Design review of the part built by this model. Coordinates are the model's own, in mm. A direction names the side the tool comes from. Round coordinates to 2 decimals unless told otherwise and drop trailing zeros. Write each loop counter-clockwise with the first axis right and the second up, starting at its lowest first coordinate (ties: lowest second). Pieces come first, ordered by that corner, then holes. Notation, with made-up numbers: M -25,17.25 L -16,17.25 A5 cw -16,23.25 Z; hole C 65,59 d11. An arc over 180 degrees is marked long. One line per question, with ' | ' between items. Start each with the question number.
Item 1: For L1, parallel to Y at x = -69.4, z = 7.75; L2, parallel to X at y = 15, z = 5.5; L3, parallel to Y at x = -69.4, z = 4, list the stretches that pass through material, from the lowest coordinate up.
Item 2: Add section B-B, the plane y = 30.8. State the section outline as (x, z) points, and give its area (3 significant figures).
Item 3: Insertion check: pin 1 Ø11 at (x, y) = (-46, 21) entering from -Z; pin 2 Ø2 at (x, z) = (-47, 9.5) entering from -Y; pin 3 Ø1 at (x, z) = (-60.5, 5.5) entering from -Y. Each pin has a flat end and moves straight along its axis. Give the tip position at first contact, or say it passes through.
Item 4: Machinability: for faces 4 (the face through (-49, 5, 13)), 5 (the face through (-66.231, -31, 7)), 6 (the face through (-38, 14.75, 5)), 7 (the face through (-61, 26.3, 11)), which of the approach directions +Z, -Z, +X, -X, +Y, -Y give a long, thin tool a straight path to every point of the face, cutting with its end or side? Answer none if there is none.
Item 5: Add section A-A, the plane y = -21. State the section outline as (x, z) points, and give its area (3 significant figures).
Item 6: Add section D-D, the plane z = 0.5. State the section outline as (x, y) points, and give its area (3 significant figures).
Item 7: Draft analysis for pull direction X (two halves, no side actions). For faces 1 (the face through (-70, 13.5, 3)), 2 (the face through (-46.05, 13.76, 0.27)), 3 (the face through (-52, 26, 7.5)), state which applies: released by +X, released by -X, zero draft, split by the parting line, or undercut.
Item 8: Add section C-C, the plane x = -47.5. State the section outline as (y, z) points.
```python
from build123d import *

# Parameters (mm, degrees)
SKETCH009_W     = 40
SKETCH009_H     = 69
SKETCH009_R     = 1.75
SKETCH009_W_2   = 31.3
SKETCH009_H_2   = 57.6
PAD004_DEPTH    = 11
SKETCH010_W     = 28
SKETCH010_H     = 23
POCKET005_DEPTH = 8
SKETCH011_W     = 28
SKETCH011_H     = 5
POCKET006_DEPTH = 8
SKETCH012_W     = 25
SKETCH012_H     = 3
POCKET007_DEPTH = 7
SKETCH013_W     = 38
SKETCH013_H     = 5.5
POCKET008_DEPTH = 5
SKETCH014_W     = 31.3
SKETCH014_H     = 2
PAD005_DEPTH    = 11
SKETCH015_W     = 12.5
SKETCH015_H     = 3
POCKET009_DEPTH = 5
SKETCH016_W     = 38
SKETCH016_H     = 5.5
POCKET010_DEPTH = 23.5
PAD006_DEPTH    = 23.5
SKETCH018_W     = 1.2
SKETCH018_H     = 38
PAD007_DEPTH    = 4.3
SKETCH019_W     = 12.15
SKETCH019_H     = 26
PAD008_DEPTH    = 1.2
SKETCH032_W     = 2.35
SKETCH032_H     = 7
POCKET014_DEPTH = 13
SKETCH033_W     = 31.3
SKETCH033_H     = 5
PAD018_DEPTH    = 1.2
SKETCH034_R     = 12
SKETCH034_R_2   = 11
PAD019_DEPTH    = 5.5
PAD020_DEPTH    = 3.5
FILLET_R        = 3
FILLET001_R     = 1


with BuildPart() as part:
    # Sketch009 → Pad004 (new body)
    with BuildSketch(Plane.XY):
        with Locations((-0.1, -1)):
            Rectangle(SKETCH009_W, SKETCH009_H)
        with Locations((-17.5, -32.71)):
            Circle(SKETCH009_R, mode=Mode.SUBTRACT)
        with Locations((17.5, -32.71)):
            Circle(SKETCH009_R, mode=Mode.SUBTRACT)
        with Locations((-17.5, 29.8)):
            Circle(SKETCH009_R, mode=Mode.SUBTRACT)
        with Locations((17.5, 29.8)):
            Circle(SKETCH009_R, mode=Mode.SUBTRACT)
        with Locations((-0.1, -1)):
            Rectangle(SKETCH009_W_2, SKETCH009_H_2, mode=Mode.SUBTRACT)
    extrude(amount=PAD004_DEPTH)

    # Sketch010 (on Face3 of Pad004) → Pocket005 (cut)
    with BuildSketch(Plane.XZ.offset(35.5)):
        with Locations((-0.331047, 5.882488)):
            Rectangle(SKETCH010_W, SKETCH010_H)
    extrude(amount=-POCKET005_DEPTH, mode=Mode.SUBTRACT)

    # Sketch011 (on Face1 of Pocket005) → Pocket006 (cut)
    with BuildSketch(Plane(origin=(0, 33.5, 0), x_dir=(-1, 0, 0), z_dir=(0, 1, 0))):
        with Locations((0, 2.5)):
            Rectangle(SKETCH011_W, SKETCH011_H)
    extrude(amount=-POCKET006_DEPTH, mode=Mode.SUBTRACT)

    # Sketch012 (on Face9 of Pocket006) → Pocket007 (cut)
    with BuildSketch(Plane(origin=(-20.1, 0, 0), x_dir=(0, -1, 0), z_dir=(-1, 0, 0))):
        with Locations((0, 1.5)):
            Rectangle(SKETCH012_W, SKETCH012_H)
    extrude(amount=-POCKET007_DEPTH, mode=Mode.SUBTRACT)

    # Sketch013 (on Face9 of Pocket007) → Pocket008 (cut)
    with BuildSketch(Plane(origin=(-20.1, 0, 0), x_dir=(0, -1, 0), z_dir=(-1, 0, 0))):
        with Locations((-7.5, 8.25)):
            Rectangle(SKETCH013_W, SKETCH013_H)
    extrude(amount=-POCKET008_DEPTH, mode=Mode.SUBTRACT)

    # Sketch014 → Pad005 (join)
    with BuildSketch(Plane.XY):
        with Locations((-0.1, 12.75)):
            Rectangle(SKETCH014_W, SKETCH014_H)
    extrude(amount=PAD005_DEPTH)

    # Sketch015 (on Face9 of Pad005) → Pocket009 (cut)
    with BuildSketch(Plane(origin=(-20.1, 0, 0), x_dir=(0, -1, 0), z_dir=(-1, 0, 0))):
        with Locations((-6.25, 1.5)):
            Rectangle(SKETCH015_W, SKETCH015_H)
    extrude(amount=-POCKET009_DEPTH, mode=Mode.SUBTRACT)

    # Sketch016 (on Face9 of Pocket009) → Pocket010 (cut)
    with BuildSketch(Plane(origin=(-20.1, 0, 0), x_dir=(0, -1, 0), z_dir=(-1, 0, 0))):
        with Locations((-7.5, 8.25)):
            Rectangle(SKETCH016_W, SKETCH016_H)
    extrude(amount=-POCKET010_DEPTH, mode=Mode.SUBTRACT)

    # Sketch017 (on Face9 of Pocket010) → Pad006 (join)
    with BuildSketch(Plane(origin=(-20.1, 0, 0), x_dir=(0, -1, 0), z_dir=(-1, 0, 0))):
        Polygon((11.5, 11), (11.5, 5.5), (-26.5, 5.5), (-26.5, 11), (-25.3, 11), (-25.3, 6.7), (10.3, 6.7), (10.3, 11), align=None)
    extrude(amount=-PAD006_DEPTH)

    # Sketch018 (on Face45 of Pad006) → Pad007 (join)
    with BuildSketch(Plane.XY.offset(6.7)):
        with Locations((2.8, 7.5)):
            Rectangle(SKETCH018_W, SKETCH018_H)
    extrude(amount=PAD007_DEPTH)

    # Sketch019 (on Face36 of Pad007) → Pad008 (join)
    with BuildSketch(Plane(origin=(0, 0, 5.5), x_dir=(1, 0, 0), z_dir=(0, 0, -1))):
        with Locations((9.475, -13.5)):
            Rectangle(SKETCH019_W, SKETCH019_H)
    extrude(amount=-PAD008_DEPTH)

    # Sketch032 (on Face6 of Pad008) → Pocket014 (cut)
    with BuildSketch(Plane(origin=(0, 0, 0), x_dir=(1, 0, 0), z_dir=(0, 0, -1))):
        with Locations((16.725, 26.3)):
            Rectangle(SKETCH032_W, SKETCH032_H)
        with BuildLine():
            ThreePointArc((16.553467, 36.082636), (14.040903, 33.26249), (15.55, 29.8))
            Line((15.55, 29.8), (10.188963, 29.8))
            Line((10.188963, 29.8), (10.188963, 36.082636))
            Line((10.188963, 36.082636), (16.553467, 36.082636))
        make_face()
    extrude(amount=-POCKET014_DEPTH, mode=Mode.SUBTRACT)

    # Sketch033 (on Face43 of Pocket014) → Pad018 (join)
    with BuildSketch(Plane(origin=(0, 0, 5.5), x_dir=(1, 0, 0), z_dir=(0, 0, -1))):
        with Locations((-0.1, -25.3)):
            Rectangle(SKETCH033_W, SKETCH033_H)
    extrude(amount=-PAD018_DEPTH)

    # Sketch034 (on Face41 of Pad018) → Pad019 (join)
    with BuildSketch(Plane(origin=(0, 0, 5.5), x_dir=(1, 0, 0), z_dir=(0, 0, -1))):
        with Locations((-0.15, -12.83)):
            Circle(SKETCH034_R)
        with Locations((-0.15, -12.83)):
            Circle(SKETCH034_R_2, mode=Mode.SUBTRACT)
    extrude(amount=PAD019_DEPTH)

    # Sketch035 (on Face75 of Pad019) → Pad020 (join)
    with BuildSketch(Plane(origin=(0, 0, 0), x_dir=(1, 0, 0), z_dir=(0, 0, -1))):
        with BuildLine():
            ThreePointArc((-6.052, -11.75), (-6.149451, -12.748865), (-6.079047, -13.75))
            Line((-6.079047, -13.75), (5.779047, -13.75))
            ThreePointArc((5.779047, -13.75), (5.849451, -12.748865), (5.752, -11.75))
            Line((-6.052, -11.75), (5.752, -11.75))
        make_face()
    extrude(amount=PAD020_DEPTH)

    # Fillet
    fillet_edges = [part.edges().sort_by_distance(p)[0] for p in [
        (-14.331047, -35.5, 5.5),
    ]]
    fillet(fillet_edges, radius=FILLET_R)

    # Fillet001
    fillet001_edges = [part.edges().sort_by_distance(p)[0] for p in [
        (-14.331047, -29.8, 5.5),
    ]]
    fillet(fillet001_edges, radius=FILLET001_R)


with BuildPart() as part_1:
    # Body001 placement: moved
    add(part.part.moved(Location((-51.9, 1, 2))))


solid = part_1.part
```
Computed values:
1) L1: y = -34.5 to -33.46, -29.96 to 29.05, 32.55 to 34.5 | L2: x = -72 to -67.65, -63.99 to -62.99, -41.11 to -40.11, -36.35 to -32 | L3: y = -34.5 to -33.46, -29.96 to -11.5, 13.5 to 29.05, 32.55 to 34.5
2) outline: M -72,2 L -71.15,2 L -71.15,13 L -72,13 Z; M -67.65,2 L -65.9,2 L -65.9,7 L -37.9,7 L -37.9,2 L -36.15,2 L -36.15,13 L -67.65,13 Z; M -32.65,2 L -32,2 L -32,13 L -32.65,13 Z | area: 223 mm^2
3) pin 1: stops at z = 2 | pin 2: stops at y = 1.5 | pin 3: stops at y = 4.84
4) face 4: +Z, +X, -X, +Y, -Y | face 5: +Z, -Z, -Y | face 6: -Z | face 7: +Z, -X
5) outline: M -72,2 L -67.65,2 L -67.65,13 L -72,13 Z; M -36.35,2 L -32,2 L -32,13 L -36.35,13 Z | area: 95.7 mm^2
6) outline: M -57.98,14.75 A6 ccw -57.95,12.75 L -46.15,12.75 A6 ccw -46.12,14.75 Z | area: 23.9 mm^2
7) face 1: zero draft | face 2: released by +X | face 3: undercut
8) outline: M 1.5,7.5 L 2.73,7.5 L 2.73,2 L 3.82,2 L 3.82,7.5 L 12.75,7.5 L 12.75,-1.5 L 14.75,-1.5 L 14.75,7.5 L 23.84,7.5 L 23.84,2 L 24.93,2 L 24.93,7.5 L 28.8,7.5 L 28.8,7 L 34.5,7 L 34.5,13 L 28.8,13 L 28.8,8.7 L 14.75,8.7 L 14.75,13 L 12.75,13 L 12.75,8.7 L 1.5,8.7 Z
